```python
from build123d import *

# Parameters (mm, degrees)
F1_DEPTH = 1
F2_SCALE = 0.5
F3_SCALE = 0.75


# Not quite as in the source:
# - a feature of the source that left no trace in its solid (it failed there, or was rolled back) is left out


with BuildPart() as f1:
    # F0 (on Top) → F1 (new body)
    with BuildSketch(Plane.XY):
        with BuildLine():
            ThreePointArc((28.844410196, 8.0000000124), (23.9936976971, 9.2552536894), (20.3607601383, 12.7058823617))
            ThreePointArc((20.3607601383, 12.7058823617), (-20.765045237, 12.0338230128), (-0.9013340087, -23.9830689655))
            ThreePointArc((-0.9013340087, -23.9830689655), (0, -23.95), (0.9013340087, -23.9830689655))
            ThreePointArc((0.9013340087, -23.9830689655), (9.0104497198, -27.8773184793), (12.3, -36.25))
            Line((12.3, -36.25), (12.3, -39.6172702312))
            ThreePointArc((12.3, -39.6172702312), (10.3056584811, -46.3316877988), (4.9693653218, -50.8687327272))
            ThreePointArc((4.9693653218, -50.8687327272), (4.5085414865, -51.0611792515), (4.0402855379, -51.2347610435))
            ThreePointArc((4.0402855379, -51.2347610435), (-1.7764718202, -74.2905711056), (22, -74))
            ThreePointArc((22, -74), (25.527864045, -71.05572809), (30, -70))
            Line((30, -70), (54.9544511501, -70))
            ThreePointArc((54.9544511501, -70), (56.7505041703, -69.8373875368), (58.4881450694, -69.3548387097))
            ThreePointArc((58.4881450694, -69.3548387097), (85.0000000049, -30.9999999956), (58.488145074, 7.3548387217))
            ThreePointArc((58.488145074, 7.3548387217), (56.7505041744, 7.837387549), (54.9544511536, 8.0000000124))
            Line((54.9544511536, 8.0000000124), (28.844410196, 8.0000000124))
        make_face()
        with BuildLine():
            ThreePointArc((52.1479989309, -16.652173913), (60.5, -31), (52.1479989309, -45.347826087))
            ThreePointArc((52.1479989309, -45.347826087), (50.9557931419, -45.8342078169), (49.6789083458, -46))
            Line((49.6789083458, -46), (36.5, -46))
            ThreePointArc((36.5, -46), (32.9644660941, -44.5355339059), (31.5, -41))
            Line((31.5, -41), (31.5, -21))
            ThreePointArc((31.5, -21), (32.9644660941, -17.4644660941), (36.5, -16))
            Line((36.5, -16), (49.6789083458, -16))
            ThreePointArc((49.6789083458, -16), (50.9557931419, -16.1657921831), (52.1479989309, -16.652173913))
        make_face(mode=Mode.SUBTRACT)
        with BuildLine():
            ThreePointArc((0.9013340087, -23.9830689655), (0, -23.95), (-0.9013340087, -23.9830689655))
            ThreePointArc((-0.9013340087, -23.9830689655), (0, -24), (0.9013340087, -23.9830689655))
        make_face()
        with BuildLine():
            ThreePointArc((4.0402855379, -51.2347610435), (4.5085414865, -51.0611792515), (4.9693653218, -50.8687327272))
            ThreePointArc((4.9693653218, -50.8687327272), (4.501778675, -51.0440133899), (4.0402855379, -51.2347610435))
        make_face()
    extrude(amount=F1_DEPTH)


with BuildPart() as f1_1:
    # F2: moved
    add(f1.part.scale(F2_SCALE))


with BuildPart() as f1_2:
    # F3: moved
    add(f1_1.part.scale(F3_SCALE))


solid = f1_2.part
```
Build history of the part. All positions in model axes, mm. A direction names the side the tool comes from. Round coordinates to 2 decimals unless told otherwise and drop trailing zeros. Loops run counter-clockwise (first coordinate to the right, second up) from the corner with the lowest first, then second, coordinate; pieces in that order, holes last. Notation, with made-up numbers: M 31,71.25 L 60,71.25 A18 ccw 60,91.25 Z; hole C -28,60.25 d2. An arc over 180 degrees is marked long. Answer as CSV lines item,"result".
1. Two-plate mould, pull along Y, no slides. Class faces 1 (the cylindrical face through (9.02, 3.46, 0.18)), 2 (the cylindrical face through (12.38, -16.72, 0.18)), 3 (the cylindrical face through (31.873, -11.885, 0.185)), 4 (the flat face through (11, -10, 0)): released by +Y, released by -Y, zero draft, split by the parting line, or undercut.
Resolved:
face 1,"released by +Y"
face 2,"undercut"
face 3,"split by the parting line"
face 4,"zero draft"
2. 3-axis set-ups, long thin cutter, end or side, ignore diameter. For faces 5 (the cylindrical face through (12.35, -6.56, 0.18)), 6 (the cylindrical face through (9.551, -26.657, 0.185)), 7 (the cylindrical face through (3.346, -10.419, 0.185)): which of +Z, -Z, +X, -X, +Y, -Y reach the whole face in a straight line?
Resolved:
face 5,"+Z, -Z"
face 6,"+Z, -Z, +X, -Y"
face 7,"+Z, -Z, -X"
3. Wall check: probe 1 along Y at (x, z) = (18, 0.15); probe 2 along Y at (x, z) = (2, 0.2); probe 3 along X at (y, z) = (-7, 0.1). Give the ranges that are in metal, low to high. Write a range as [from, to].
Resolved:
probe 1,"y = [-26.25, -17.25], [-6, 3]"
probe 2,"y = [-29.72, -19.01], [-9.44, 8.77]"
probe 3,"x = [-5.66, 12.03], [20.61, 31.16]"
4. Cut at C-C on x = 3.75. Write the cut outline in (y, z) (3 decimals).
Resolved:
outline,"M -30,0 L -17.542,0 L -17.542,0.375 L -30,0.375 Z; M -10.908,0 L 8.182,0 L 8.182,0.375 L -10.908,0.375 Z"
5. Cut at A-A on x = 15. Write the cut outline in (y, z) (3 decimals).
Resolved:
outline,"M -26.25,0 L -17.25,0 L -17.25,0.375 L -26.25,0.375 Z; M -6,0 L 3,0 L 3,0.375 L -6,0.375 Z"
6. Cut at D-D on y = -25. Write the cut outline in (x, z) (3 decimals), then the cut area to 3 significant figures.
Resolved:
outline,"M -1.84,0 L 24.083,0 L 24.083,0.375 L -1.84,0.375 Z"
area,"9.72 mm²"
